Study the drawing (mm; zero at the part's minimum x, y, z) and answer. A direction names the side the tool comes from. Give positions to 0.01 mm unless a question says otherwise; leave off trailing zeros. Write each loop counter-clockwise with the first axis right and the second up, starting at its lowest first coordinate (ties: lowest second). Pieces come first, ordered by that corner, then holes.
1) Given pin 1 Ø5 at (x, z) = (22.5, 26) entering from -Y; pin 2 Ø6.5 at (x, z) = (4, 21) entering from -Y; pin 3 Ø6.5 at (x, y) = (8.5, 30) entering from -Z; pin 4 Ø6.5 at (x, y) = (6, 23) entering from +Z, each flat-ended and moving along its own axis, determine where each tip first touches the part or whether it passes through.
2) Find section A-A (z = 25.4). Determine the outline of the cut face in (x, y).
3) Find section B-B (x = 38.1). Determine the outline of the cut face in (y, z), plus the area to 3 significant figures.
4) Straight lines are drawn through the part: probe 1 along Z at (x, y) = (38, 30); probe 2 along X at (y, z) = (7.5, 25) (1 decimal); probe 3 along X at (y, z) = (29, 25) (1 decimal). For each, find the intervals that lie inside material, in ascending order.
5) A tool of negligible diameter and unlimited length cuts with its end or side. For the marked faces 4, 5 and 6, from which of +Z, -Z, +X, -X, +Y, -Y can it reach the whole face along a straight path? Write none if from no direction.
6) Find section C-C (y = 25.4). Determine the outline of the cut face in (x, z).
7) Find section D-D (x = 6.5). Determine the outline of the cut face in (y, z).
8) Determine the mould class of the marked faces 1, 2 and 3 for opening direction Z: pulls with the +Z half, pulls with the -Z half, needs draft (parallel to the pull), parting line crosses it, or undercut.
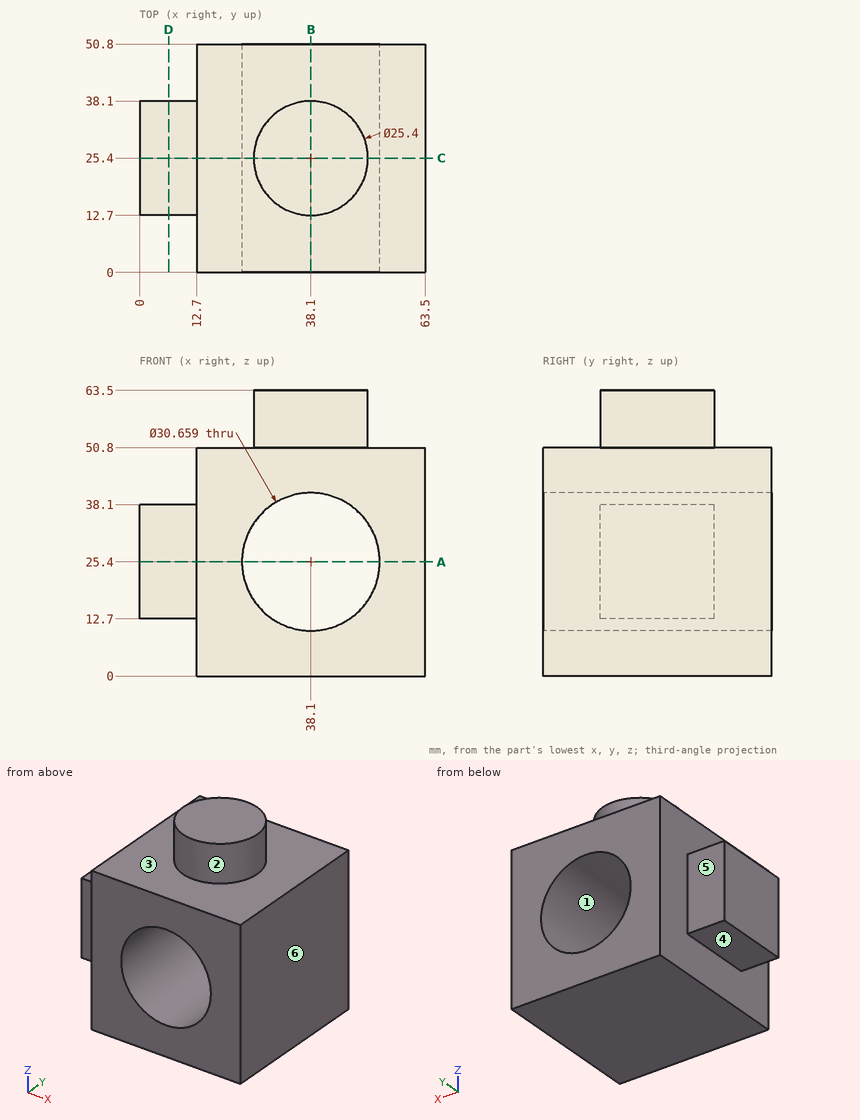
Results:
1. pin 1: stops at y = 0
1. pin 2: stops at y = 12.7
1. pin 3: stops at z = 12.7
1. pin 4: stops at z = 38.1
2. outline: (0, 12.7) - (12.7, 12.7) - (12.7, 0) - (22.77, 0) - (22.77, 50.8) - (12.7, 50.8) - (12.7, 38.1) - (0, 38.1) - close; (53.43, 0) - (63.5, 0) - (63.5, 50.8) - (53.43, 50.8) - close
3. outline: (0, 0) - (50.8, 0) - (50.8, 10.07) - (0, 10.07) - close; (0, 40.73) - (50.8, 40.73) - (50.8, 50.8) - (38.1, 50.8) - (38.1, 63.5) - (12.7, 63.5) - (12.7, 50.8) - (0, 50.8) - close
3. area: 1,350 mm2
4. probe 1: z = 0 to 10.07, 40.73 to 63.5
4. probe 2: x = 12.7 to 22.8, 53.4 to 63.5
4. probe 3: x = 0 to 22.8, 53.4 to 63.5
5. face 4: -Z, -X, +Y, -Y
5. face 5: +Z, -Z, -X, +Y
5. face 6: +Z, -Z, +X, +Y, -Y
6. outline: (0, 12.7) - (12.7, 12.7) - (12.7, 0) - (63.5, 0) - (63.5, 50.8) - (50.8, 50.8) - (50.8, 63.5) - (25.4, 63.5) - (25.4, 50.8) - (12.7, 50.8) - (12.7, 38.1) - (0, 38.1) - close; hole circle Ø30.66 at (38.1, 25.4)
7. outline: (12.7, 12.7) - (38.1, 12.7) - (38.1, 38.1) - (12.7, 38.1) - close
8. face 1: undercut
8. face 2: needs draft
8. face 3: pulls with the +Z half
